Check sheet for the drawn part. Datum: minimum x, y, z corner. Units: mm. A direction names the side the tool comes from. Coordinates: 2 decimals unless noted, no trailing zeros. Loops run counter-clockwise (first coordinate to the right, second up) from the corner with the lowest first, then second, coordinate; pieces in that order, holes last. Notation, with made-up numbers: M -35.5,81 L -3.5,81 A31 cw -3.5,110 Z; hole C -29,26 d8. An arc over 180 degrees is marked long. Answer in a Markdown table with one row per item. Add a question column.
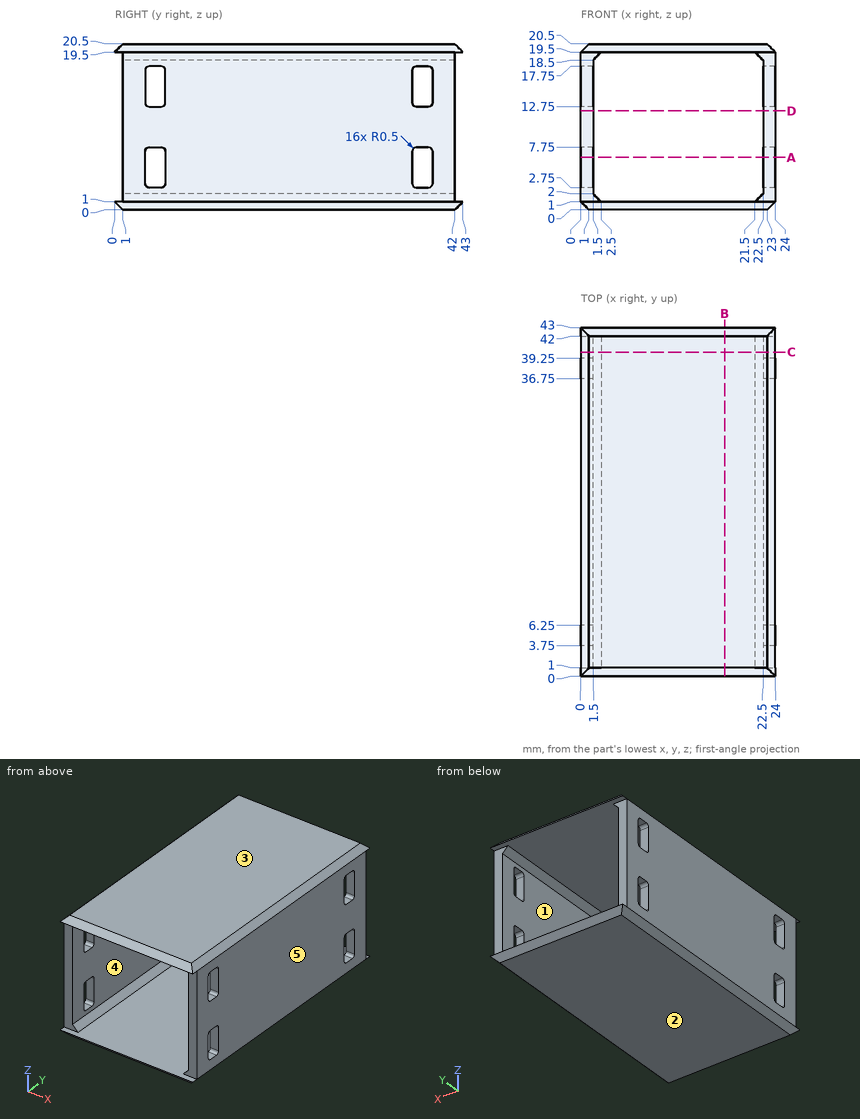
Q1. Cross-section at B-B (x = 17.75). Record the cut outline in (y, z), plus the area to 3 significant figures.
Q2. Go/stop test with flat-tipped pins: pin 1 (1.6 mm diameter, centred on x = 1, z = 14.5, fed in from -Y); pin 2 (1.3 mm diameter, centred on x = 22.5, z = 14, fed in from +Y); pin 3 (2 mm diameter, centred on x = 21, z = 15.5, fed in from -Y). Record where each tip stops, or that it passes through.
Q3. Mould release check, pull along X, two halves, no side actions. Record for the marked faces 3, 4 and 5: released by +X, released by -X, zero draft, split by the parting line, or undercut.
Q4. Thickness scan on L1, parallel to Z at x = 8.5, y = 18.5; L2, parallel to X at y = 22.5, z = 8; L3, parallel to Z at x = 22.25, y = 18. Record the ranges inside material, lowest first.
Q5. Cross-section at A-A (z = 6.5). Record the cut outline in (x, y).
Q6. Access from +Z, -Z, +X, -X, +Y, -Y to the whole of each face (thin tool, end or side, straight path). Record for the marked faces 1 and 2.
Q7. Cross-section at D-D (z = 12.25). Record the cut outline in (x, y).
Q8. Cross-section at C-C (y = 40). Record the cut outline in (x, z).
Answer key:
| question | item | result |
|---|---|---|
| 1 | outline | M 0,1 L 1,0 L 42,0 L 43,1 Z; M 0,19.5 L 43,19.5 L 42,20.5 L 1,20.5 Z |
| 1 | area | 84.0 mm^2 |
| 2 | pin 1 | y = 1 |
| 2 | pin 2 | y = 42 |
| 2 | pin 3 | through |
| 3 | face 3 | zero draft |
| 3 | face 4 | undercut |
| 3 | face 5 | released by +X |
| 4 | L1 | 0 to 1, 19.5 to 20.5 |
| 4 | L2 | 0 to 1.5, 22.5 to 24 |
| 4 | L3 | 0 to 1.75, 18.75 to 20.5 |
| 5 | outline | M 0,1 L 1.5,1 L 1.5,3.75 L 0,3.75 Z; M 0,6.25 L 1.5,6.25 L 1.5,36.75 L 0,36.75 Z; M 0,39.25 L 1.5,39.25 L 1.5,42 L 0,42 Z; M 22.5,1 L 24,1 L 24,3.75 L 22.5,3.75 Z; M 22.5,6.25 L 24,6.25 L 24,36.75 L 22.5,36.75 Z; M 22.5,39.25 L 24,39.25 L 24,42 L 22.5,42 Z |
| 6 | face 1 | +Y, -Y |
| 6 | face 2 | -Z, +X, -X, +Y, -Y |
| 7 | outline | M 0,1 L 1.5,1 L 1.5,42 L 0,42 Z; M 22.5,1 L 24,1 L 24,42 L 22.5,42 Z |
| 8 | outline | M 0,1 L 1,0 L 23,0 L 24,1 L 24,19.5 L 23,20.5 L 1,20.5 L 0,19.5 Z; hole M 1.5,2 L 2.5,1 L 21.5,1 L 22.5,2 L 22.5,18.5 L 21.5,19.5 L 2.5,19.5 L 1.5,18.5 Z |
